Can you work these out from the model? Positions are in its coordinate system, mm. A direction names the side the tool comes from. Give positions to 0.01 mm unless a question says otherwise; leave off trailing zeros. Order: outer loops, then holes, each group sorted by start corner. A loop starts at its lowest first (then second) coordinate and runs counter-clockwise, first axis right, second up. Notation, with made-up numbers: (29.25, -32.5) - (52.25, -32.5) arc R18 ccw to (52.25, -12.5) - close; hole circle Ø3 at (12, 37). An arc over 180 degrees is marked (long way). Answer as CSV lines item,"result".
Autodesk Fusion 360 part; units mm, degrees
sketch "Sketch1" plane through (0, 0, 0) normal (0, 1, 0) x (1, 0, 0)
  line L0 (0, 0) -> (10, 0)
  line L1 (5, 0) -> (5, 10)
  line L2 (0, 0) -> (0, 15)
  line L3 (0, 15) -> (10, 15)
  line L4 (10, 15) -> (10, 0)
  circle A0 centre (5, 10) radius 1.5
  dimension "d1" = 3
extrude "Extrude1" add sketch "Sketch1" along normal blind 5
sketch "Sketch2" plane through (0, 0, 0) normal (0, 0, 1) x (1, 0, 0)
  line L0 (0, 0) -> (10, 0)
  line L1 (10, 0) -> (10, 5)
  line L2 (10, 5) -> (0, 5)
  line L3 (0, 5) -> (0, 0)
  line L4 (5, 0) -> (5, 10)
  line L5 (0, 5) -> (0, 15)
  line L6 (0, 15) -> (10, 15)
  line L7 (10, 15) -> (10, 5)
  circle A0 centre (5, 10) radius 1.5
  dimension "d4" = 10
  dimension "d5" = 3
extrude "Extrude2" add sketch "Sketch2" against normal blind 5 contours L2 L5 L6 L7
fillet "Fillet1" radius 2 4 edges at (10, 15, -2.5) (10, 2.5, -15) (0, 15, -2.5) (0, 2.5, -15)
1) I'm going to push flat-ended pins straight in: P1, Ø5, axis at x = 5, y = 10, coming from the -Z side; P2, Ø3, axis at x = 8, z = -6.5, coming from the -Y side; P3, Ø1.8, axis at x = 5, z = -10, coming from the +Y side; P4, Ø3, axis at x = 5, z = -8.5, coming from the +Y side. Where does each tip first touch, or does it pass through?
Answer block:
P1,"z = -5"
P2,"y = 0"
P3,"through"
P4,"y = 5"
2) I want a section at C-C on x = 5. Write out the boundary of the cut face in (y, z).
Answer block:
outline,"(0, -15) - (5, -15) - (5, -11.5) - (0, -11.5) - close; (0, -8.5) - (5, -8.5) - (5, -5) - (8.5, -5) - (8.5, 0) - (0, 0) - close; (11.5, -5) - (15, -5) - (15, 0) - (11.5, 0) - close"
3) Which directions (+Z, -Z, +X, -X, +Y, -Y) give clear straight access to the entire face, cutting with the end or side of a thin tool? Please do faces 4 (the flat face through (0, 5, -4)), 5 (the flat face through (3.8, 11.2, -5)).
Answer block:
face 4,"+Z, -Z, -X, +Y, -Y"
face 5,"-Z, +X, -X, +Y"
4) If we mould it in two halves opening along Y, with no side actions, what happens to faces 1 (the flat face through (3.8, 5, -11.2)), 2 (the cylindrical face through (6.386, 9.425, -2.465)), 3 (the flat face through (5, 7, 0))? For each: +Y half, -Y half, draft (parallel to the pull), parting line (faces both ways), or undercut.
Answer block:
face 1,"+Y half"
face 2,"undercut"
face 3,"draft"
5) I want a section at D-D on z = -10. Write out the boundary of the cut face in (x, y).
Answer block:
outline,"(0, 0) - (3.5, 0) - (3.5, 5) - (0, 5) - close; (6.5, 0) - (10, 0) - (10, 5) - (6.5, 5) - close"
6) I want a section at B-B on y = 10. Write out the boundary of the cut face in (x, z).
Answer block:
outline,"(0, -5) - (3.5, -5) - (3.5, 0) - (0, 0) - close; (6.5, -5) - (10, -5) - (10, 0) - (6.5, 0) - close"
7) I want a section at A-A on z = -4. Write out the boundary of the cut face in (x, y), plus the area to 3 significant figures.
Answer block:
outline,"(0, 0) - (10, 0) - (10, 13) arc R2 ccw to (8, 15) - (2, 15) arc R2 ccw to (0, 13) - close; hole circle Ø3 at (5, 10)"
area,"141 mm2"
8) I need wall thicknesses on line 1 along Y through (x, z) = (5, -3.85); line 2 along X through (y, z) = (10, -3.05); line 3 along Z through (x, y) = (5, 2.9). Which ranges of each line are inside material? Lowest first, please. Write a range as [from, to].
Answer block:
line 1,"[0, 8.5], [11.5, 15]"
line 2,"[0, 3.5], [6.5, 10]"
line 3,"[-15, -11.5], [-8.5, 0]"
